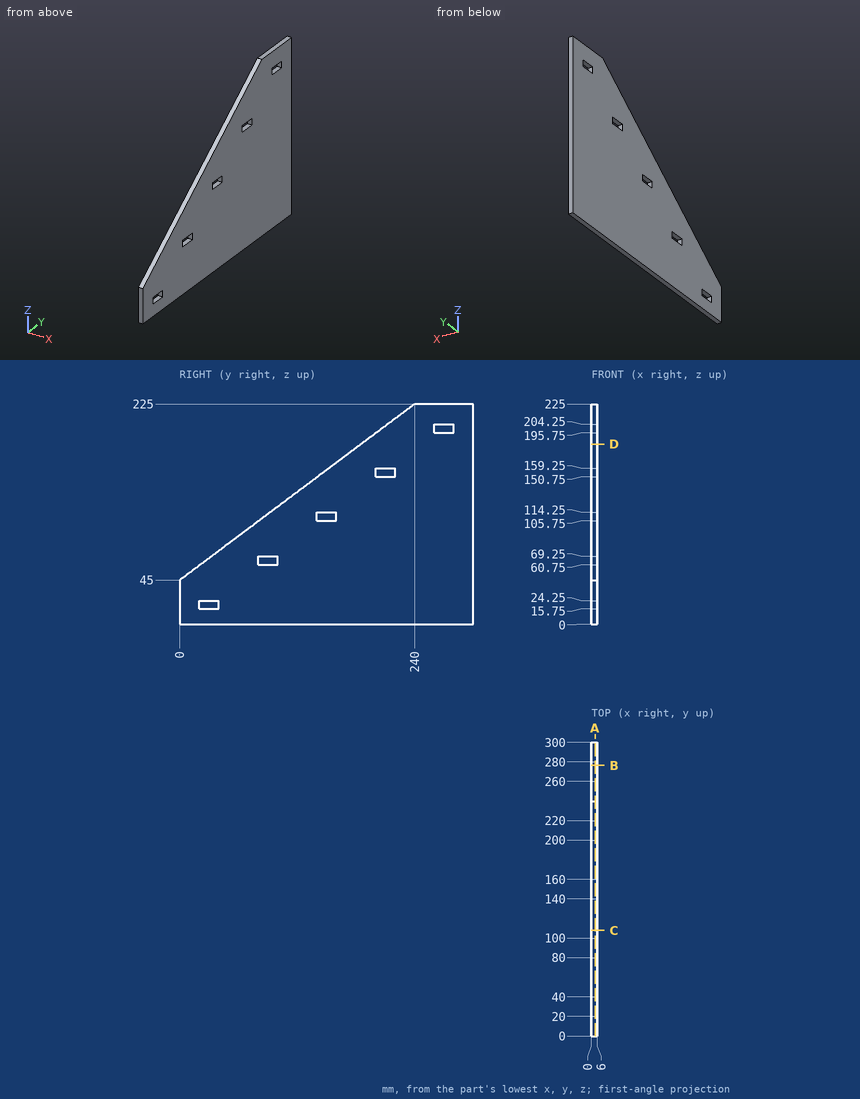
Study the drawing (mm; zero at the part's minimum x, y, z) and answer. Give positions to 0.01 mm unless a question says otherwise; leave off trailing zeros. Loops run counter-clockwise (first coordinate to the right, second up) from the corner with the lowest first, then second, coordinate; pieces in that order, holes last. Notation, with made-up numbers: (66.25, 30) -> (75.25, 30) arc R27 cw to (75.25, 64) -> close; hole circle Ø2 at (-33.75, -0.75). An arc over 180 degrees is marked (long way). Use a Markdown table: item, result. Add a question column.
1) The part is cut by section A-A, the plane x = 3.9. Determine the outline of the cut face in (y, z).
2) The part is cut by section B-B, the plane y = 276.5. Determine the outline of the cut face in (x, z).
3) Each of these flat-tipped pins is pushed along its axis until it touches: P1, Ø1.5, axis at x = 2, z = 70.5, coming from the -Y side; P2, Ø1.8, axis at x = 3, y = 205, coming from the +Z side (3 decimals); P3, Ø3, axis at x = 1.5, y = 147.5, coming from the +Z side; P4, Ø1.8, axis at x = 2, y = 207.5, coming from the -Z side. Where does it stop, or does it pass through?
4) The part is cut by section D-D, the plane z = 184. Determine the outline of the cut face in (x, y), plus the area to 3 significant figures.
5) The part is cut by section C-C, the plane y = 108. Determine the outline of the cut face in (x, z).
6) Consider line 1 along Z through (x, y) = (5.5, 268); line 2 along Y through (x, z) = (1.2, 20.5); line 3 along Z through (x, y) = (2.85, 23.5) (3 decimals). Determine where each line is inside the solid, lowest interval first.
Reported:
| question | item | result |
|---|---|---|
| 1 | outline | (0, 0) -> (300, 0) -> (300, 225) -> (240, 225) -> (0, 45) -> close; hole (20, 15.75) -> (40, 15.75) -> (40, 24.25) -> (20, 24.25) -> close; hole (80, 60.75) -> (100, 60.75) -> (100, 69.25) -> (80, 69.25) -> close; hole (140, 105.75) -> (160, 105.75) -> (160, 114.25) -> (140, 114.25) -> close; hole (200, 150.75) -> (220, 150.75) -> (220, 159.25) -> (200, 159.25) -> close; hole (260, 195.75) -> (280, 195.75) -> (280, 204.25) -> (260, 204.25) -> close |
| 2 | outline | (0, 0) -> (6, 0) -> (6, 195.75) -> (0, 195.75) -> close; (0, 204.25) -> (6, 204.25) -> (6, 225) -> (0, 225) -> close |
| 3 | P1 | stops at y = 33 |
| 3 | P2 | stops at z = 199.425 |
| 3 | P3 | stops at z = 156.75 |
| 3 | P4 | stops at z = 0 |
| 4 | outline | (0, 185.33) -> (6, 185.33) -> (6, 300) -> (0, 300) -> close |
| 4 | area | 688 mm^2 |
| 5 | outline | (0, 0) -> (6, 0) -> (6, 126) -> (0, 126) -> close |
| 6 | line 1 | z = 0 to 195.75, 204.25 to 225 |
| 6 | line 2 | y = 0 to 20, 40 to 300 |
| 6 | line 3 | z = 0 to 15.75, 24.25 to 62.625 |
